The figure shows three views and two pictorial views of one solid part (mm, origin at its lowest corner). Answer the questions. A direction names the side the tool comes from. Give positions to 0.01 mm unless a question says otherwise; leave off trailing zeros. Loops run counter-clockwise (first coordinate to the right, second up) from the corner with the lowest first, then second, coordinate; pieces in that order, holes last. Notation, with made-up numbers: M -1,82 L 46,82 A26 cw 46,99 Z; hole C 27.25,38 d1. An arc over 180 degrees is marked long. Write item = value, one per line. Start each with the question number.
1. Flat-ended cylindrical pins translate along their axes: pin 1 Ø1.2 at (x, y) = (14.5, 6.5) entering from +Z; pin 2 Ø1.2 at (x, z) = (1.5, 4) entering from -Y; pin 3 Ø1.6 at (y, z) = (9.5, 4) entering from +X; pin 4 Ø3 at (x, z) = (4, 3) entering from +Y. Find the tip coordinate at first contact, or state that the pin passes through.
2. Section A-A on z = 5.5 is taken. Determine the outline of the cut face in (x, y), plus the area to 3 significant figures.
3. Section C-C on x = 9.5 is taken. Determine the outline of the cut face in (y, z), plus the area to 3 significant figures.
4. Section B-B on y = 11.5 is taken. Determine the outline of the cut face in (x, z).
5. The mould has two halves that part along X. Classify the marked faces 1, 2 and 3: released by +X, released by -X, zero draft, split by the parting line, or undercut.
6. For the marked faces 4, 5, 6, 7 and 8, determine the directions among +Z, -Z, +X, -X, +Y, -Y from which every point of the face is accessible in a straight line to the end or side of a thin tool.
7. Consider L1, parallel to Z at x = 12.25, y = 13; L2, parallel to Z at x = 14, y = 8; L3, parallel to X at y = 14, z = 4. Determine where each line is inside the solid, lowest interval first. Write a range as [from, to].
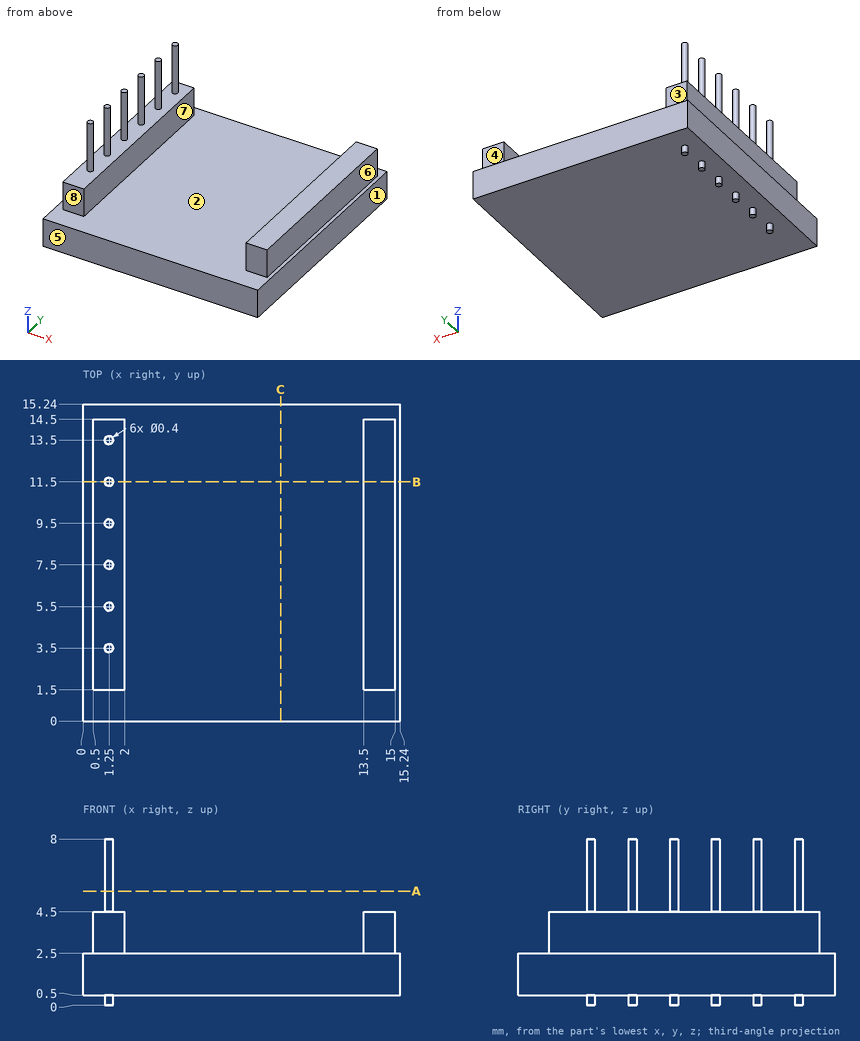
Verdict:
q1.pin_1 = 4.5
q1.pin_2 = 1.5
q1.pin_3 = 15
q1.pin_4 = 15.24
q2.outline = C 1.25,3.5 d0.4; C 1.25,5.5 d0.4; C 1.25,7.5 d0.4; C 1.25,9.5 d0.4; C 1.25,11.5 d0.4; C 1.25,13.5 d0.4
q2.area = 0.754 mm2
q3.outline = M 0,0.5 L 15.24,0.5 L 15.24,2.5 L 0,2.5 Z
q3.area = 30.5 mm2
q4.outline = M 0,0.5 L 1.05,0.5 L 1.05,0 L 1.45,0 L 1.45,0.5 L 15.24,0.5 L 15.24,2.5 L 15,2.5 L 15,4.5 L 13.5,4.5 L 13.5,2.5 L 2,2.5 L 2,4.5 L 1.45,4.5 L 1.45,8 L 1.05,8 L 1.05,4.5 L 0.5,4.5 L 0.5,2.5 L 0,2.5 Z
q5.face_1 = released by +X
q5.face_2 = undercut
q5.face_3 = zero draft
q6.face_4 = +Z, +X, -X, +Y
q6.face_5 = +Z, -Z, +X, -X, -Y
q6.face_6 = +Z, +X, +Y, -Y
q6.face_7 = +Z, +Y, -Y
q6.face_8 = +Z, +X, -X, -Y
q7.L1 = [0.5, 2.5]
q7.L2 = [0.5, 4.5]
q7.L3 = [0.5, 2], [13.5, 15]
